Autodesk Inventor part; units mm, degrees
ref_plane "YZ Plane" through (0, 0, 0) normal (1, 0, 0) x (0, 1, 0)
ref_plane "XZ Plane" through (0, 0, 0) normal (0, 1, 0) x (-1, 0, 0)
ref_plane "XY Plane" through (0, 0, 0) normal (0, 0, 1) x (1, 0, 0)
sketch "Sketch1" plane through (0, 0, 0) normal (0, 0, 1) x (1, 0, 0)
  line L0 (-19.8053, 20.7004) -> (-19.8053, -11.0496)
  line L1 (-19.8053, -11.0496) -> (30.9947, -11.0496)
  line L2 (30.9947, -11.0496) -> (30.9947, 1.6504)
  line L3 (30.9947, 1.6504) -> (-7.1053, 1.6504)
  line L4 (-7.1053, 1.6504) -> (-7.1053, 20.7004)
  line L5 (-7.1053, 20.7004) -> (-19.8053, 20.7004)
  point P0 (0, 0)
  dimension "d0" = 12.7
  dimension "d1" = 50.8
  dimension "d2" = 12.7
  dimension "d3" = 31.75
extrude "Extrusion1" add sketch "Sketch1" along normal blind 31.75
sketch "Sketch2" plane through (-7.1053, 1.6504, 0) normal (1, 0, 0) x (0, 0, -1)
  line L0 (0, 19.05) -> (-31.75, 19.05)
  line L1 (-25.4, 19.05) -> (-6.35, 19.05)
  line L2 (-6.35, 19.05) -> (-6.35, 12.7)
  line L3 (-6.35, 12.7) -> (-25.4, 12.7)
  line L4 (-25.4, 12.7) -> (-25.4, 19.05)
  line L5 (-31.75, 0) -> (-31.75, 19.05)
  line L6 (0, 0) -> (0, 19.05)
  point P0 (0, -1.6504)
  dimension "d6" = 6.35
  dimension "d7" = 6.35
  dimension "d8" = 6.35
extrude "Extrusion2" cut sketch "Sketch2" against normal blind 31.75
sketch "Sketch3" plane through (-7.1053, 1.6504, 0) normal (0, 1, 0) x (1, 0, 0)
  line L0 (38.1, 0) -> (38.1, -31.75)
  line L1 (38.1, -22.225) -> (12.7, -22.225)
  line L2 (12.7, -22.225) -> (12.7, -9.525)
  line L3 (12.7, -9.525) -> (38.1, -9.525)
  line L4 (38.1, -9.525) -> (38.1, -22.225)
  line L5 (-12.7, 0) -> (38.1, 0)
  line L6 (38.1, -31.75) -> (0, -31.75)
  point P0 (7.1053, 0)
  dimension "d11" = 9.525
  dimension "d12" = 9.525
  dimension "d13" = 25.4
extrude "Extrusion3" cut sketch "Sketch3" against normal blind 31.75
properties part number "Figure 7_27_1"
Here's how the part is built. I have some questions about the finished solid (model axes, mm). A direction names the side the tool comes from. Round coordinates to 2 decimals unless told otherwise and drop trailing zeros. Loops run counter-clockwise (first coordinate to the right, second up) from the corner with the lowest first, then second, coordinate; pieces in that order, holes last. Notation, with made-up numbers: (-15.75, 71.5) - (10.25, 71.5) arc R17 cw to (10.25, 82.5) - close; hole circle Ø11 at (19.25, -24.75). An arc over 180 degrees is marked (long way). One line per question, with ' | ' between items. Start each with the question number.
Q1. Please list where these lines run through material, in increasing order: line 1 (Z direction, x = 25, y = 1.5) (3 decimals); line 2 (Y direction, x = 15, z = 4.5); line 3 (X direction, y = -5, z = 11). Write a range as [from, to].
Q2. We'd pull the mould along Z, two halves only. Please class faces 5 (the flat face through (5, -11.05, 16)), 6 (the flat face through (0, -2, 31.75)), 7 (the flat face through (-13, 14.35, 16)): +Z half, -Z half, draft (parallel to the pull), parting line (faces both ways), or undercut.
Q3. I want a section at D-D (x = -14). Write out the boundary of the cut face in (y, z), then the cut area to 3 significant figures.
Q4. For faces 1 (the flat face through (5.595, -5, 16)), 2 (the flat face through (-7.105, 9, 16)), 3 (the flat face through (-13, 20.7, 3)), 4 (the flat face through (-13, 17, 25.4)), which set-ups out of +Z, -Z, +X, -X, +Y, -Y let a thin tool reach every point of the face, with its end or its side?
Q5. I want a section at A-A (x = 17.5). Write out the boundary of the cut face in (y, z) (3 decimals).
Q6. I want a section at C-C (z = 16). Write out the boundary of the cut face in (x, y), then the cut area to 3 significant figures.
Q7. I want a section at B-B (y = 18). Write out the boundary of the cut face in (x, z), then the cut area to 3 significant figures.
Q8. Will these pins go through, and if not, where does the flat tip stop? pin 1 (3 mm diameter, centred on x = 4, z = 26.5, fed in from +Y); pin 2 (5.5 mm diameter, centred on y = 15.5, z = 12.5, fed in from +X); pin 3 (1 mm diameter, centred on x = 7.5, z = 11.5, fed in from -Y).
Response values:
1) line 1: z = [0, 9.525], [22.225, 31.75] | line 2: y = [-11.05, 1.65] | line 3: x = [-19.81, 5.59]
2) face 5: draft | face 6: +Z half | face 7: undercut
3) outline: (-11.05, 0) - (20.7, 0) - (20.7, 6.35) - (14.35, 6.35) - (14.35, 25.4) - (20.7, 25.4) - (20.7, 31.75) - (-11.05, 31.75) - close | area: 887 mm²
4) face 1: +X, +Y, -Y | face 2: +Z, -Z, +X, +Y | face 3: +Z, -Z, +X, -X, +Y | face 4: +X, -X, +Y
5) outline: (-11.05, 0) - (1.65, 0) - (1.65, 9.525) - (-11.05, 9.525) - close; (-11.05, 22.225) - (1.65, 22.225) - (1.65, 31.75) - (-11.05, 31.75) - close
6) outline: (-19.81, -11.05) - (5.59, -11.05) - (5.59, 1.65) - (-7.11, 1.65) - (-7.11, 14.35) - (-19.81, 14.35) - close | area: 484 mm²
7) outline: (-19.81, 0) - (-7.11, 0) - (-7.11, 6.35) - (-19.81, 6.35) - close; (-19.81, 25.4) - (-7.11, 25.4) - (-7.11, 31.75) - (-19.81, 31.75) - close | area: 161 mm²
8) pin 1: stops at y = 1.65 | pin 2: stops at x = -7.11 | pin 3: passes through
